Build history of the part. All positions in model axes, mm. Face numbers are marked on the shaded views. A direction names the side the tool comes from. Coordinates: 2 decimals unless noted, no trailing zeros. Write each loop counter-clockwise with the first axis right and the second up, starting at its lowest first coordinate (ties: lowest second). Pieces come first, ordered by that corner, then holes. Notation, with made-up numbers: (47, 81) -> (73, 81) arc R27 ccw to (73, 108) -> close; hole circle Ø1 at (-15, 5.25). An arc over 180 degrees is marked (long way). Write each question's results on one line, items separated by ' | '. Start each with the question number.
Q1. Saw through at C-C on z = 0. Give the cut face in (x, y), and give its area (3 significant figures).
Q2. Saw through at D-D on y = -0.5. Give the cut face in (x, z), and give its area (3 significant figures).
Q3. Drop flat-ended pins along their axis: pin 1 Ø4 at (y, z) = (-6.5, 8.5) entering from +X; pin 2 Ø8 at (x, z) = (0, 0) entering from +Y; pin 3 Ø8 at (x, z) = (0, 0.5) entering from +Y; pin 4 Ø1.2 at (y, z) = (-2.5, 0.5) entering from +X. Give the stop position or say it passes through.
Q4. Drill centre lines: line 1 (Y direction, x = 0, z = 7.4); line 2 (Z direction, x = 0, y = -2.45); line 3 (X direction, y = 15, z = 5.9). Where is each one in solid material? Low to high.
Q5. Two-plate mould, pull along Y, no slides. Class the marked faces 1, 2 and 3: released by +Y, released by -Y, zero draft, split by the parting line, or undercut.
Q6. Saw through at B-B on y = 8.5. Give the cut face in (x, z), and give its area (3 significant figures).
Q7. Tool access for the marked faces 4, 5, 6 and 7: list every direction of +Z, -Z, +X, -X, +Y, -Y with a clear straight run to the whole face (end or side of a thin tool).
Q8. Saw through at A-A on z = -6. Give the cut face in (x, y), and give its area (3 significant figures).
from build123d import *

# Parameters (mm, degrees)
BOX007_W              = 11
BOX007_H              = 7
BOX007_DEPTH          = 10
FILLET_R              = 3
ARRAY_COUNT           = 2
ARRAY_ANGLE           = 180
ARRAY_PLACEMENT_ANGLE = 90
CYLINDER004_R         = 3
CYLINDER004_DEPTH     = 30
CYLINDER_R            = 3.5
CYLINDER_DEPTH        = 15
CYLINDER006_R         = 6
CYLINDER006_DEPTH     = 4
CYLINDER005_R         = 6
CYLINDER005_DEPTH     = 4
BOX001_W              = 5
BOX001_H              = 10
BOX001_DEPTH          = 5
BOX002_W              = 20
BOX002_H              = 25
BOX002_DEPTH          = 5
BOX_W                 = 20
BOX_H                 = 5
BOX_DEPTH             = 20
FILLET001_R           = 9.9
FILLET002_R           = 2
CHAMFER_SIZE          = 1
CHAMFER001_SIZE       = 0.5


with BuildPart() as array:
    # Box007 → Box007 (new body)
    with BuildSketch(Plane(origin=(10, 5, -5), x_dir=(1, 0, 0), z_dir=(0, 0, 1))):
        with Locations((5.5, 3.5)):
            Rectangle(BOX007_W, BOX007_H)
    extrude(amount=BOX007_DEPTH)


with BuildPart() as array_1:
    # BaseFeature placement: moved
    add(array.part.moved(Location((-10, -5, 5))))

    # Fillet
    fillet_edges = [array_1.edges().sort_by_distance(p)[0] for p in [
        (5.5, 0, 10),
        (5.5, 0, 0),
    ]]
    fillet(fillet_edges, radius=FILLET_R)


with BuildPart() as array_2:
    # Body placement: moved
    add(array_1.part.moved(Location((-5, 5, 0))))

    # Array: Array ×2 about axis
    array_axis = Axis((0, 0, 0), (0, 0, 1))


with BuildPart() as array_3:
    add(array_2.part)
    for i in range(1, ARRAY_COUNT):
        add(array_2.part.rotate(array_axis, i * ARRAY_ANGLE / (ARRAY_COUNT - 1)))


with BuildPart() as array_4:
    # Array placement: moved
    add(array_3.part.moved(Location((0, -3, -5))).rotate(Axis((0, -3, -5), (0, 0, 1)), ARRAY_PLACEMENT_ANGLE))


with BuildPart() as cilindro004:
    # Cylinder004 → Cylinder004 (new body)
    with BuildSketch(Plane(origin=(0, 15, -15), x_dir=(1, 0, 0), z_dir=(0, 0, 1))):
        Circle(CYLINDER004_R)
    extrude(amount=CYLINDER004_DEPTH)


with BuildPart() as cilindro:
    # Cylinder → Cylinder (new body)
    with BuildSketch(Plane.XZ.offset(-5)):
        Circle(CYLINDER_R)
    extrude(amount=CYLINDER_DEPTH)


with BuildPart() as obj1:
    # Cylinder006 → Cylinder006 (new body)
    with BuildSketch(Plane.XY.offset(4.3)):
        Circle(CYLINDER006_R)
    extrude(amount=CYLINDER006_DEPTH)


with BuildPart() as fusion003:
    # Cylinder005 → Cylinder005 (new body)
    with BuildSketch(Plane.XY.offset(-8.3)):
        Circle(CYLINDER005_R)
    extrude(amount=CYLINDER005_DEPTH)

    # Fusion003: union obj1
    add(obj1.part)


with BuildPart() as fusion003_1:
    # Fusion003 placement: moved
    add(fusion003.part.moved(Location((0, 15, 0))))


with BuildPart() as pin0:
    # Box001 → Box001 (new body)
    with BuildSketch(Plane(origin=(-2.5, -10, 5), x_dir=(1, 0, 0), z_dir=(0, 0, 1))):
        with Locations((2.5, 5)):
            Rectangle(BOX001_W, BOX001_H)
    extrude(amount=BOX001_DEPTH)


with BuildPart() as pin001:
    # Clone base: copy of pin0
    add(pin0.part)


with BuildPart() as pin001_1:
    # Clone placement: moved
    add(pin001.part.moved(Location((0, 0, -15))))


with BuildPart() as pared1:
    # Box002 → Box002 (new body)
    with BuildSketch(Plane(origin=(-10, 0, 5), x_dir=(1, 0, 0), z_dir=(0, 0, 1))):
        with Locations((10, 12.5)):
            Rectangle(BOX002_W, BOX002_H)
    extrude(amount=BOX002_DEPTH)


with BuildPart() as pared002:
    # Clone001 base: copy of pared1
    add(pared1.part)


with BuildPart() as pared002_1:
    # Clone001 placement: moved
    add(pared002.part.moved(Location((0, 0, -15))))


with BuildPart() as chamfer001001:
    # Box → Box (new body)
    with BuildSketch(Plane(origin=(-10, -5, -10), x_dir=(1, 0, 0), z_dir=(0, 0, 1))):
        with Locations((10, 2.5)):
            Rectangle(BOX_W, BOX_H)
    extrude(amount=BOX_DEPTH)

    # Fusion: union pin0, pin001, pared1, pared002
    add(pin0.part)
    add(pin001_1.part)
    add(pared1.part)
    add(pared002_1.part)

    # Fusion004: union Fusion003
    add(fusion003_1.part)

    # Cut001: cut Cilindro
    add(cilindro.part, mode=Mode.SUBTRACT)

    # Cut002: cut Cilindro004
    add(cilindro004.part, mode=Mode.SUBTRACT)

    # Cut003: cut Array
    add(array_4.part, mode=Mode.SUBTRACT)

    # Fillet001
    fillet001_edges = [chamfer001001.edges().sort_by_distance(p)[0] for p in [
        (10, 25, -7.5),
        (10, 25, 7.5),
        (-10, 25, 7.5),
        (-10, 25, -7.5),
    ]]
    fillet(fillet001_edges, radius=FILLET001_R)

    # Fillet002
    fillet002_edges = [chamfer001001.edges().sort_by_distance(p)[0] for p in [
        (-10, 5.05, -10),
        (-10, 5.05, 10),
    ]]
    fillet(fillet002_edges, radius=FILLET002_R)

    # Chamfer
    chamfer_edges = [chamfer001001.edges().sort_by_distance(p)[0] for p in [
        (-3.5, 0, 0),
    ]]
    chamfer(chamfer_edges, length=CHAMFER_SIZE)

    # Chamfer001
    chamfer001_edges = [chamfer001001.edges().sort_by_distance(p)[0] for p in [
        (-6, 15, -4.3),
        (-6, 15, 4.3),
    ]]
    chamfer(chamfer001_edges, length=CHAMFER001_SIZE)


solid = chamfer001001.part
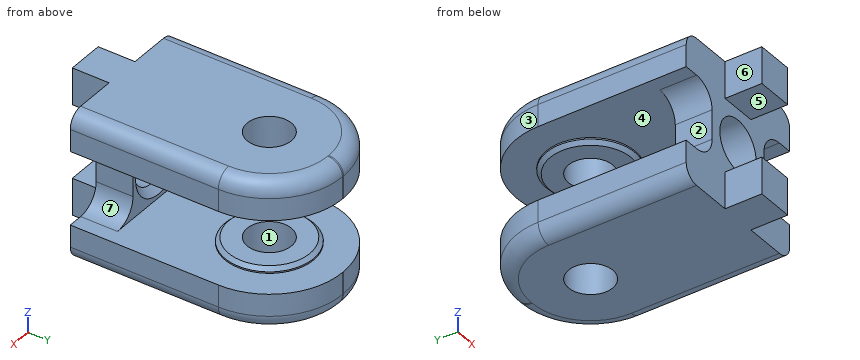
Returned:
1) outline: (-5, -5) -> (-3.5, -5) -> (-3.5, -1) -> (-4.5, 0) -> (-5, 0) -> close; (3.5, -5) -> (5, -5) -> (5, 0) -> (4.5, 0) -> (3.5, -1) -> close | area: 14.0 mm2
2) outline: (-10, -8) arc R2 ccw to (-8, -10) -> (8, -10) arc R2 ccw to (10, -8) -> (10, -5) -> (8, -5) arc R3 cw to (5, -2) -> (5, 2) arc R3 cw to (8, 5) -> (10, 5) -> (10, 8) arc R2 ccw to (8, 10) -> (-8, 10) arc R2 ccw to (-10, 8) -> (-10, 5) -> (-8, 5) arc R3 cw to (-5, 2) -> (-5, -2) arc R3 cw to (-8, -5) -> (-10, -5) -> close; hole circle Ø8 at (0, 0) | area: 254 mm2
3) pin 1: stops at x = 10 | pin 2: stops at y = -0.5 | pin 3: stops at y = 20.7 | pin 4: stops at x = 5
4) line 1: y = -10 to 12, 18 to 25 | line 2: z = -10 to -3.5, 3.5 to 10 | line 3: x = -10 to -3, 3 to 10
5) face 1: undercut | face 2: zero draft | face 3: released by +Y
6) outline: (-10, -8) arc R2 ccw to (-8, -10) -> (8, -10) arc R2 ccw to (10, -8) -> (10, -5) -> (-10, -5) -> close; (-10, 5) -> (10, 5) -> (10, 8) arc R2 ccw to (8, 10) -> (-8, 10) arc R2 ccw to (-10, 8) -> close | area: 197 mm2
7) face 4: none | face 5: +X, -X, -Y | face 6: +Z, -Z, -X, -Y | face 7: +X, +Y, -Y
8) outline: (-10, -5) -> (-2.5, -5) -> (-2.5, -10) -> (2.5, -10) -> (2.5, -5) -> (10, -5) -> (10, 15.1) arc R9.9 ccw to (0.1, 25) -> (-0.1, 25) arc R9.9 ccw to (-10, 15.1) -> close; hole circle Ø6 at (0, 15) | area: 555 mm2
